Here's how the part is built. I have some questions about the finished solid (model axes, mm). Face numbers are marked on the shaded views. A direction names the side the tool comes from. Round coordinates to 2 decimals unless told otherwise and drop trailing zeros. Loops run counter-clockwise (first coordinate to the right, second up) from the corner with the lowest first, then second, coordinate; pieces in that order, holes last. Notation, with made-up numbers: (58.25, -29.5) -> (114.25, -29.5) arc R21 cw to (114.25, 3.5) -> close; hole circle Ø4 at (71.25, 57). An arc over 180 degrees is marked (long way). One line per item, written item: value. Start each with the question number.
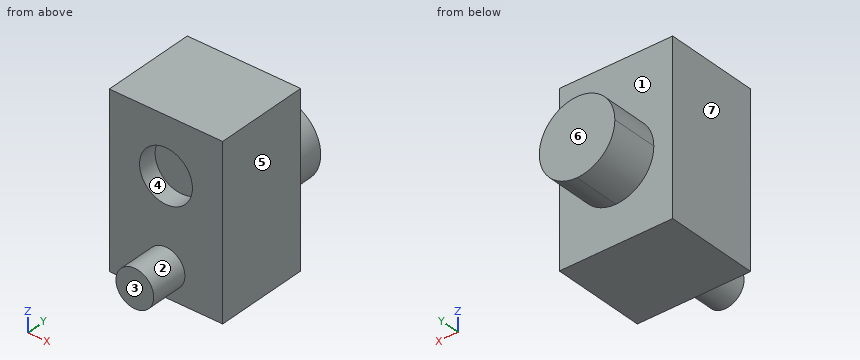
```python
from build123d import *

# Parameters (mm, degrees)
F0_W     = 60
F0_H     = 60
F1_DEPTH = 90
F2_DEPTH = 10
F4_DEPTH = 25
F5_W     = 60
F5_H     = 90
F5_R     = 10
F6_DEPTH = 20
F7_R     = 14
F8_DEPTH = 10


with BuildPart() as f1:
    # F0 (on Top) → F1 (new body)
    with BuildSketch(Plane.XY):
        Rectangle(F0_W, F0_H)
    extrude(amount=F1_DEPTH)

    # F2 (add): a face of the model
    f2_faces = [f1.faces().sort_by_distance(p)[0] for p in [
        (0, -30, 45),
    ]]
    extrude(f2_faces, amount=F2_DEPTH)

    # F3 (on face) → F4 (join)
    with BuildSketch(Plane(origin=(0, 30, 0), x_dir=(-1, 0, 0), z_dir=(0, 1, 0))):
        with BuildLine():
            ThreePointArc((0, 20), (14.1421356237, 25.8578643763), (20, 40))
            ThreePointArc((20, 40), (-14.1421356237, 54.1421356237), (0, 20))
        make_face()
    extrude(amount=F4_DEPTH)

    # F5 (on face) → F6 (cut)
    with BuildSketch(Plane.XZ.offset(40)):
        with Locations((0, 45)):
            Rectangle(F5_W, F5_H)
        with Locations((0, 15)):
            Circle(F5_R, mode=Mode.SUBTRACT)
    extrude(amount=-F6_DEPTH, mode=Mode.SUBTRACT)

    # F7 (on face) → F8 (cut)
    with BuildSketch(Plane.XZ.offset(20)):
        with Locations((0, 60)):
            Circle(F7_R)
    extrude(amount=-F8_DEPTH, mode=Mode.SUBTRACT)


solid = f1.part
```
Q1. If I drill on line 1 along Z through (x, y) = (0, -15); line 2 along Y through (x, z) = (10, 62); line 3 along Y through (x, z) = (-20.5, 12.5), over which ranges is the centre line in solid material (lowest first)?
Q2. I want a section at D-D on z = 58.5. Please give me the cut outline in (x, y), plus the area to 3 significant figures.
Q3. If we mould it in two halves opening along X, with no side actions, what happens to the marked faces 4, 5, 6 and 7? For each: released by +X, released by -X, zero draft, split by the parting line, or undercut.
Q4. I want a section at C-C on y = 40. Please give me the cut outline in (x, z), plus the area to 3 significant figures.
Q5. Which directions (+Z, -Z, +X, -X, +Y, -Y) give clear straight access to the entire face, cutting with the end or side of a thin tool? Please do the marked faces 1, 2 and 3.
Q6. I want a section at B-B on x = -3.5. Please give me the cut outline in (y, z), plus the area to 3 significant figures.
Q7. Will these pins go through, and if not, where does the flat tip stop? P1, Ø10, axis at x = 1, z = 45.5, coming from the -Y side; P2, Ø5, axis at y = 43.5, z = 54, coming from the -X side; P3, Ø25, axis at x = 0, z = 60, coming from the -Y side.
Q8. I want a section at A-A on z = 15. Please give me the cut outline in (x, y).
Answers below:
1. line 1: z = 0 to 46, 74 to 90
1. line 2: y = -10 to 30
1. line 3: y = -20 to 30
2. outline: (-30, -20) -> (-13.92, -20) -> (-13.92, -10) -> (13.92, -10) -> (13.92, -20) -> (30, -20) -> (30, 30) -> (7.6, 30) -> (7.6, 55) -> (-7.6, 55) -> (-7.6, 30) -> (-30, 30) -> close
2. area: 3,100 mm^2
3. face 4: undercut
3. face 5: released by +X
3. face 6: zero draft
3. face 7: released by -X
4. outline: circle Ø40 at (0, 40)
4. area: 1,260 mm^2
5. face 1: +Y
5. face 2: -Y
5. face 3: +Z, -Z, +X, -X, -Y
6. outline: (-40, 5.63) -> (-20, 5.63) -> (-20, 0) -> (30, 0) -> (30, 20.31) -> (55, 20.31) -> (55, 59.69) -> (30, 59.69) -> (30, 90) -> (-20, 90) -> (-20, 73.56) -> (-10, 73.56) -> (-10, 46.44) -> (-20, 46.44) -> (-20, 24.37) -> (-40, 24.37) -> close
6. area: 5,590 mm^2
7. P1: stops at y = -20
7. P2: stops at x = -16.36
7. P3: stops at y = -10
8. outline: (-30, -20) -> (-10, -20) -> (-10, -40) -> (10, -40) -> (10, -20) -> (30, -20) -> (30, 30) -> (-30, 30) -> close
